Can you work these out from the model? Positions are in its coordinate system, mm. A direction names the side the tool comes from. Give positions to 0.01 mm unless a question says otherwise; leave off trailing zeros. Loops run counter-clockwise (first coordinate to the right, second up) from the corner with the lowest first, then second, coordinate; pieces in that order, holes last.
from build123d import *

# Parameters (mm, degrees)
F0_W     = 127
F0_H     = 127
F1_DEPTH = 127
F3_DEPTH = 101.6


# Not quite as in the source:
# - a feature names something its author has since deleted; it is built from what else it names


with BuildPart() as f1:
    # F0 (on Top) → F1 (new body)
    with BuildSketch(Plane.XY):
        Rectangle(F0_W, F0_H)
    extrude(amount=-F1_DEPTH)

    # F2 (on Top) → F3 (cut)
    with BuildSketch(Plane.XY):
        Polygon((-12.9577365428, 63.5224819239), (-63.7577365428, 63.5224819239), (-63.7577365428, 12.7224819239), align=None)
        Polygon((12.7373517871, -63.3020326495), (63.5373517871, -63.3020326495), (63.5373517871, -12.5020326495), align=None)
    extrude(amount=-F3_DEPTH, mode=Mode.SUBTRACT)


solid = f1.part
(1) Will these pins go through, and if not, where does the flat tip stop? P1, Ø10, axis at x = -39.5, z = -33, coming from the +Y side; P2, Ø5, axis at y = -50, z = -68.5, coming from the +X side.
Returned:
P1: stops at y = 41.98
P2: stops at x = 28.54
(2) Suppose I cut it at C-C on y = 26. List the corners of the cut face in (x, z) for me, plus the area to 3 significant figures.
Returned:
outline: (-63.5, -127) - (63.5, -127) - (63.5, 0) - (-50.48, 0) - (-50.48, -101.6) - (-63.5, -101.6) - close
area: 14,800 mm2
(3) Thinking about a two-plate mould opening in Y: for faces 4 (the flat face through (-1, 1, 0)), 5 (the flat face through (49, -49, -101.6)), 6 (the flat face through (13, 63.5, -77)), which applies, pulls with the +Y half, pulls with the -Y half, needs draft (parallel to the pull), parting line crosses it, or undercut?
Returned:
face 4: needs draft
face 5: undercut
face 6: pulls with the +Y half
(4) Which directions (+Z, -Z, +X, -X, +Y, -Y) give clear straight access to the entire face, cutting with the end or side of a thin tool? Please do faces 1 (the flat face through (-1, 1, -127)), 2 (the flat face through (38.47, -37.57, -50.09)), 3 (the flat face through (-44, 44, -101.6)).
Returned:
face 1: -Z, +X, -X, +Y, -Y
face 2: +Z, +X
face 3: +Z, -X, +Y
(5) Suppose I cut it at B-B on x = 36. List the corners of the cut face in (y, z) for me.
Returned:
outline: (-63.5, -127) - (63.5, -127) - (63.5, 0) - (-40.04, 0) - (-40.04, -101.6) - (-63.3, -101.6) - (-63.3, 0) - (-63.5, 0) - close
(6) Please list where these lines run through material, in increasing order: probe 1 along Z at (x, y) = (30, -57.5); probe 2 along Y at (x, z) = (46, -22); probe 3 along Y at (x, z) = (-25.5, -91).
Returned:
probe 1: z = -127 to -101.6
probe 2: y = -63.5 to -63.3, -30.04 to 63.5
probe 3: y = -63.5 to 50.98
(7) Suppose I cut it at A-A on z = -21. List the corners of the cut face in (x, y) for me, plus the area to 3 significant figures.
Returned:
outline: (-63.5, -63.5) - (63.5, -63.5) - (63.5, -63.3) - (12.74, -63.3) - (63.5, -12.54) - (63.5, 63.5) - (-12.98, 63.5) - (-63.5, 12.98) - close
area: 13,600 mm2
(8) Suppose I cut it at D-D on y = -47.5. List the corners of the cut face in (x, z) for me.
Returned:
outline: (-63.5, -127) - (63.5, -127) - (63.5, -101.6) - (28.54, -101.6) - (28.54, 0) - (-63.5, 0) - close
